Source: CAD feature listing. Evaluate the final solid. Frame: model axes, mm. Face numbers are marked on the shaded views. A direction names the side the tool comes from. Round coordinates to 2 decimals unless told otherwise and drop trailing zeros. Order: outer loops, then holes, each group sorted by start corner. A loop starts at its lowest first (then second) coordinate and runs counter-clockwise, first axis right, second up. Notation, with made-up numbers: M 35.25,25 L 89.25,25 A11 ccw 89.25,46 Z; hole C 77.25,38 d6. An arc over 180 degrees is marked long. Use one line per item in the form item = value. Start each with the question number.
Q1. Section A-A (z = 29). Return the cut outline in (x, y), plus the area to 3 significant figures.
Q2. Section D-D (z = -2). Return the cut outline in (x, y).
Q3. Section B-B (y = 45). Return the cut outline in (x, z).
Q4. Material intervals for probe 1 along Y at (x, z) = (20.5, 1); probe 2 along Z at (x, y) = (15, 13.5); probe 3 along X at (y, z) = (7, 24.5), sorted ascending.
Q5. Reachability of the marked faces 4 and 5 from +Z, -Z, +X, -X, +Y, -Y: full face, straight path, thin tool, end or side. Return the list, or none.
Q6. Contact query for flat-ended pins moving along their axis: pin 1 (10 mm diameter, centred on y = 18.5, z = 43, fed in from +X); pin 2 (1.5 mm diameter, centred on x = 30, z = -31, fed in from -Y); pin 3 (4 mm diameter, centred on y = 10.5, z = 33.5, fed in from -X). Output: stop coordinate, or through.
Q7. Pull-direction query (Z, two-part tool) for the marked faces 1, 2 and 3; classes: pulls with the +Z half, pulls with the -Z half, needs draft (parallel to the pull), parting line crosses it, or undercut.
Q8. Section C-C (x = -51). Return the cut outline in (y, z), plus the area to 3 significant figures.
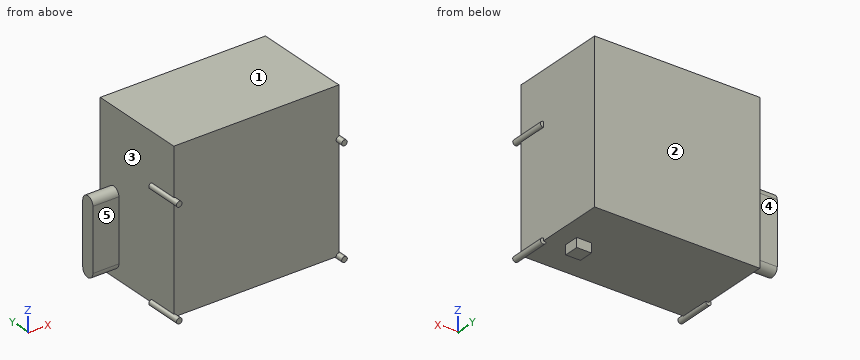
from build123d import *

# Parameters (mm, degrees)
SKETCH2_R                = 1.5
BOSS_EXTRUDE1_DEPTH      = 20
BOSS_EXTRUDE1_2_DEPTH    = 20
BOSS_EXTRUDE1_3_DEPTH    = 20
BOSS_EXTRUDE1_4_DEPTH    = 20
BOSS_EXTRUDE2_DEPTH      = 37
BOSS_EXTRUDE2_DEPTH_BACK = 16
SKETCH3_W                = 89
SKETCH3_H                = 85
BOSS_EXTRUDE5_DEPTH      = 14
SKETCH8_W                = 8
SKETCH8_H                = 8
BOSS_EXTRUDE6_DEPTH      = 5


with BuildPart() as part:
    # Sketch2 → Boss-Extrude1 (new body)
    with BuildSketch(Plane(origin=(0, 0, 0), x_dir=(1, 0, 0), z_dir=(0, 1, 0))):
        with Locations(Location((-44.5, 29, 0), (0, 0, 270))):
            Circle(SKETCH2_R)
    extrude(amount=BOSS_EXTRUDE1_DEPTH)



with BuildPart() as body_2:
    # Sketch2 → Boss-Extrude1 2 (new body)
    with BuildSketch(Plane(origin=(0, 0, 0), x_dir=(1, 0, 0), z_dir=(0, 1, 0))):
        with Locations(Location((44.5, 29, 0), (0, 0, 270))):
            Circle(SKETCH2_R)
    extrude(amount=BOSS_EXTRUDE1_2_DEPTH)


with BuildPart() as body_3:
    # Sketch2 → Boss-Extrude1 3 (new body)
    with BuildSketch(Plane(origin=(0, 0, 0), x_dir=(1, 0, 0), z_dir=(0, 1, 0))):
        with Locations(Location((-44.5, -29, 0), (0, 0, 270))):
            Circle(SKETCH2_R)
    extrude(amount=BOSS_EXTRUDE1_3_DEPTH)


with BuildPart() as body_4:
    # Sketch2 → Boss-Extrude1 4 (new body)
    with BuildSketch(Plane(origin=(0, 0, 0), x_dir=(1, 0, 0), z_dir=(0, 1, 0))):
        with Locations(Location((44.5, -29, 0), (0, 0, 270))):
            Circle(SKETCH2_R)
    extrude(amount=BOSS_EXTRUDE1_4_DEPTH)


with BuildPart() as part_1:
    add(part.part)

    add(body_2.part)  # Boss-Extrude2 merges body 2

    add(body_3.part)  # Boss-Extrude2 merges body 3

    add(body_4.part)  # Boss-Extrude2 merges body 4
    # Sketch3 → Boss-Extrude2 (add, two sides: drawn at the far end of the back side and taken through both)
    with BuildSketch(Plane(origin=(0, 20, 0), x_dir=(1, 0, 0), z_dir=(0, 1, 0)).offset(-BOSS_EXTRUDE2_DEPTH_BACK)):
        with Locations((0, -13.5)):
            Rectangle(SKETCH3_W, SKETCH3_H)
    extrude(amount=BOSS_EXTRUDE2_DEPTH + BOSS_EXTRUDE2_DEPTH_BACK)

    # Sketch7 → Boss-Extrude5 (add)
    with BuildSketch(Plane.ZY.offset(44.5)):
        with BuildLine():
            Line((-20.661260067, 50.895180513), (12.711227635, 50.895180513))
            ThreePointArc((12.711227635, 50.895180513), (16.370214945, 47.236193203), (12.711227635, 43.577205894))
            Line((12.711227635, 43.577205894), (-20.661260067, 43.577205894))
            ThreePointArc((-20.661260067, 43.577205894), (-24.320247376, 47.236193203), (-20.661260067, 50.895180513))
        make_face()
    extrude(amount=BOSS_EXTRUDE5_DEPTH)

    # Sketch8 → Boss-Extrude6 (add)
    with BuildSketch(Plane(origin=(0, 0, -29), x_dir=(-1, 0, 0), z_dir=(0, 0, -1))):
        with Locations((-30.8, 27.15)):
            Rectangle(SKETCH8_W, SKETCH8_H)
    extrude(amount=BOSS_EXTRUDE6_DEPTH)


solid = part_1.part
Results list:
q1.outline = M -46,0 L -43,0 L -43,4 L 43,4 L 43,0 L 46,0 L 46,20 L 44.5,20 L 44.5,57 L -44.5,57 L -44.5,20 L -46,20 Z
q1.area = 4,790 mm2
q2.outline = M -58.5,43.58 L -44.5,43.58 L -44.5,4 L 44.5,4 L 44.5,57 L -44.5,57 L -44.5,50.9 L -58.5,50.9 Z
q3.outline = M -58.5,-23.56 L -44.5,-23.56 L -44.5,-29 L 44.5,-29 L 44.5,56 L -44.5,56 L -44.5,15.61 L -58.5,15.61 Z
q4.probe_1 = 4 to 57
q4.probe_2 = -29 to 56
q4.probe_3 = -44.5 to 44.5
q5.face_4 = +Z, -Z, -X, +Y
q5.face_5 = +Z, -Z, -X, -Y
q6.pin_1 = 44.5
q6.pin_2 = 23.15
q6.pin_3 = -44.5
q7.face_1 = pulls with the +Z half
q7.face_2 = needs draft
q7.face_3 = undercut
q8.outline = M 43.58,-20.66 A3.66 ccw 50.9,-20.66 L 50.9,12.71 A3.66 ccw 43.58,12.71 Z
q8.area = 286 mm2
